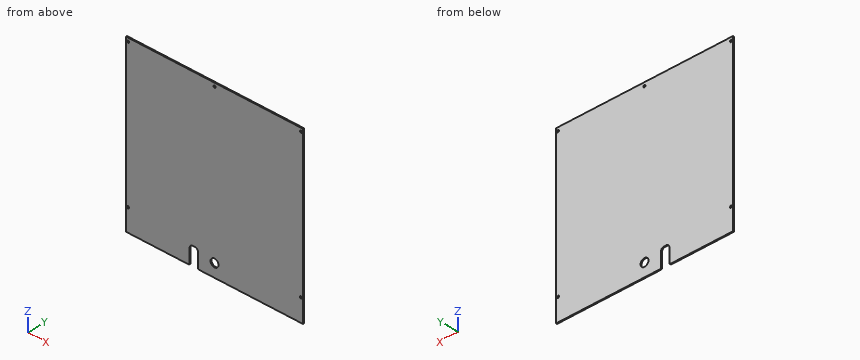
from build123d import *

# Parameters (mm, degrees)
CROQUIS12_W           = 335
CROQUIS12_H           = 329.4
BRIDA_BASE2_DEPTH     = 2
CORTAR_EXTRUIR6_REACH = 269.058
CROQUIS27_R           = 2
CORTAR_EXTRUIR7_REACH = 269.058
CROQUIS28_R           = 7.5
CROQUIS29_W           = 16
CROQUIS29_H           = 35
CORTAR_EXTRUIR8_DEPTH = 268.058214815
REDONDEO1_R           = 6
REDONDEO2_R           = 2


# Sheet-metal steps are written as plain solids
with BuildPart() as part:
    # Croquis12 → Brida base2 (new body)
    with BuildSketch(Plane(origin=(0, 0, 0), x_dir=(1, 0, 0), z_dir=(0, 1, 0))):
        with Locations((0, -43.29)):
            Rectangle(CROQUIS12_W, CROQUIS12_H)
    extrude(amount=-BRIDA_BASE2_DEPTH)

    # Croquis27 → Cortar-Extruir6 (cut, up to next)
    with BuildSketch(Plane(origin=(0, 0, 0), x_dir=(1, 0, 0), z_dir=(0, 1, 0)), mode=Mode.PRIVATE) as cortar_extruir6_sk1:
        with Locations(Location((-163.7, -201.3, 0), (0, 0, 270))):
            Circle(CROQUIS27_R)
    cortar_extruir6_tool1 = extrude(cortar_extruir6_sk1.sketch, amount=-CORTAR_EXTRUIR6_REACH, mode=Mode.PRIVATE) & part.part
    # Croquis27 → Cortar-Extruir6 (cut, up to next)
    with BuildSketch(Plane(origin=(0, 0, 0), x_dir=(1, 0, 0), z_dir=(0, 1, 0)), mode=Mode.PRIVATE) as cortar_extruir6_sk2:
        with Locations(Location((-163.7, 78.26, 0), (0, 0, 270))):
            Circle(CROQUIS27_R)
    cortar_extruir6_tool2 = extrude(cortar_extruir6_sk2.sketch, amount=-CORTAR_EXTRUIR6_REACH, mode=Mode.PRIVATE) & part.part
    # Croquis27 → Cortar-Extruir6 (cut, up to next)
    with BuildSketch(Plane(origin=(0, 0, 0), x_dir=(1, 0, 0), z_dir=(0, 1, 0)), mode=Mode.PRIVATE) as cortar_extruir6_sk3:
        with Locations(Location((163.7, 78.26, 0), (0, 0, 90))):
            Circle(CROQUIS27_R)
    cortar_extruir6_tool3 = extrude(cortar_extruir6_sk3.sketch, amount=-CORTAR_EXTRUIR6_REACH, mode=Mode.PRIVATE) & part.part
    # Croquis27 → Cortar-Extruir6 (cut, up to next)
    with BuildSketch(Plane(origin=(0, 0, 0), x_dir=(1, 0, 0), z_dir=(0, 1, 0)), mode=Mode.PRIVATE) as cortar_extruir6_sk4:
        with Locations(Location((163.7, -201.3, 0), (0, 0, 90))):
            Circle(CROQUIS27_R)
    cortar_extruir6_tool4 = extrude(cortar_extruir6_sk4.sketch, amount=-CORTAR_EXTRUIR6_REACH, mode=Mode.PRIVATE) & part.part
    # Croquis27 → Cortar-Extruir6 (cut, up to next)
    with BuildSketch(Plane(origin=(0, 0, 0), x_dir=(1, 0, 0), z_dir=(0, 1, 0)), mode=Mode.PRIVATE) as cortar_extruir6_sk5:
        with Locations(Location((0, -201.3, 0), (0, 0, 270))):
            Circle(CROQUIS27_R)
    cortar_extruir6_tool5 = extrude(cortar_extruir6_sk5.sketch, amount=-CORTAR_EXTRUIR6_REACH, mode=Mode.PRIVATE) & part.part
    add(cortar_extruir6_tool1.solids().sort_by_distance((-163.7, 0, 201.3))[0], mode=Mode.SUBTRACT)
    add(cortar_extruir6_tool2.solids().sort_by_distance((-163.7, 0, -78.26))[0], mode=Mode.SUBTRACT)
    add(cortar_extruir6_tool3.solids().sort_by_distance((163.7, 0, -78.26))[0], mode=Mode.SUBTRACT)
    add(cortar_extruir6_tool4.solids().sort_by_distance((163.7, 0, 201.3))[0], mode=Mode.SUBTRACT)
    add(cortar_extruir6_tool5.solids().sort_by_distance((0, 0, 201.3))[0], mode=Mode.SUBTRACT)

    # Croquis28 → Cortar-Extruir7 (cut, up to next)
    with BuildSketch(Plane(origin=(0, 0, 0), x_dir=(1, 0, 0), z_dir=(0, 1, 0)), mode=Mode.PRIVATE) as cortar_extruir7_sk1:
        with Locations(Location((0, 96.25, 0), (0, 0, 270))):
            Circle(CROQUIS28_R)
    cortar_extruir7_tool1 = extrude(cortar_extruir7_sk1.sketch, amount=-CORTAR_EXTRUIR7_REACH, mode=Mode.PRIVATE) & part.part
    add(cortar_extruir7_tool1.solids().sort_by_distance((0, 0, -96.25))[0], mode=Mode.SUBTRACT)

    # Croquis29 → Cortar-Extruir8 (cut, through all)
    with BuildSketch(Plane(origin=(0, 0, 0), x_dir=(1, 0, 0), z_dir=(0, 1, 0))):
        with Locations((-39, 103.91)):
            Rectangle(CROQUIS29_W, CROQUIS29_H)
    extrude(amount=-CORTAR_EXTRUIR8_DEPTH, mode=Mode.SUBTRACT)

    # Redondeo1
    redondeo1_edges = [part.edges().sort_by_distance(p)[0] for p in [
        (-47, -1, -86.41),
        (-31, -1, -86.41),
    ]]
    fillet(redondeo1_edges, radius=REDONDEO1_R)

    # Redondeo2
    redondeo2_edges = [part.edges().sort_by_distance(p)[0] for p in [
        (-47, -1, -121.41),
        (-31, -1, -121.41),
    ]]
    fillet(redondeo2_edges, radius=REDONDEO2_R)


solid = part.part
Build history of the part. All positions in model axes, mm. Coordinates: 2 decimals unless noted, no trailing zeros. Order: outer loops, then holes, each group sorted by start corner. A loop starts at its lowest first (then second) coordinate and runs counter-clockwise, first axis right, second up. Notation, with made-up numbers: (23.5, 16.25) -> (43.5, 16.25) arc R22 ccw to (43.5, 22.25) -> close; hole circle Ø5 at (29, -30.75). An arc over 180 degrees is marked (long way). One line per item, written item: value.
(1) Slice it at A-A, the plane z = -96.25. List the corners of the cut face in (x, y).
Checked values:
outline: (-167.5, -2) -> (-47, -2) -> (-47, 0) -> (-167.5, 0) -> close; (-31, -2) -> (-7.5, -2) -> (-7.5, 0) -> (-31, 0) -> close; (7.5, -2) -> (167.5, -2) -> (167.5, 0) -> (7.5, 0) -> close
(2) Drop flat-ended pins along their axis: pin 1 Ø2.5 at (x, z) = (-163.7, -78.26) entering from -Y; pin 2 Ø1 at (x, y) = (-39.5, -1) entering from -Z. Give the stop position or say it passes through.
Checked values:
pin 1: through
pin 2: z = -86.41
(3) Probe line 1 (X direction, y = -0.6, z = -78.26); line 2 (Z direction, x = 163.7, y = -1.35); line 3 (X direction, y = -1.5, z = 201.3). List the from-to ranges inside material, lowest first. Write a range as [from, to].
Checked values:
line 1: [-167.5, -165.7], [-161.7, 161.7], [165.7, 167.5]
line 2: [-121.41, -80.26], [-76.26, 199.3], [203.3, 207.99]
line 3: [-167.5, -165.7], [-161.7, -2], [2, 161.7], [165.7, 167.5]
